```python
from build123d import *

# Parameters (mm, degrees)
BASE_FLANGE1_DEPTH                           = 19.5
SKETCH13_R                                   = 4
CUT_EXTRUDE6_DEPTH                           = 84.228219974
CUT_EXTRUDE7_DEPTH                           = 84.228219974
CUT_EXTRUDE7_DEPTH_BACK                      = 84.228219974
SKETCH33_R                                   = 8
CUT_EXTRUDE10_DEPTH                          = 10
SKETCH34_R                                   = 1.5
CUT_EXTRUDE11_DEPTH                          = 10
BOSS_EXTRUDE1_DEPTH                          = 3
TAB1_START                                   = -3
TAB1_DEPTH                                   = 3
CSK_FOR_M4_COUNTERSUNK_FLAT_HEAD_SCR_2_COUNT = 2
CSK_FOR_M4_COUNTERSUNK_FLAT_HEAD_SCR_2_PITCH = 39.597979746
CSK_FOR_M4_COUNTERSUNK_FLAT_HEAD_SCR_3_COUNT = 2
CSK_FOR_M4_COUNTERSUNK_FLAT_HEAD_SCR_3_PITCH = 56
CSK_FOR_M4_COUNTERSUNK_FLAT_HEAD_SCR_4_COUNT = 2
CSK_FOR_M4_COUNTERSUNK_FLAT_HEAD_SCR_4_PITCH = 39.597979746
SKETCH44_R                                   = 1.25
CUT_EXTRUDE13_DEPTH                          = 10
SKETCH45_R                                   = 1.25
CUT_EXTRUDE14_DEPTH                          = 10


# Read off the part's stored shape, not the designer's step: Tab1
# Sheet-metal steps are written as plain solids
with BuildPart() as part:
    # Sketch1 → Base-Flange1 (new, symmetric)
    with BuildSketch(Plane.XY):
        with BuildLine():
            Line((-28.21, 74.65), (-28.21, 2))
            ThreePointArc((-28.21, 2), (-27.624213562, 0.585786438), (-26.21, 0))
            Line((-26.21, 0), (26.21, 0))
            ThreePointArc((26.21, 0), (27.624213562, 0.585786438), (28.21, 2))
            Line((28.21, 2), (28.21, 74.65))
            Line((28.21, 74.65), (31.21, 74.65))
            Line((31.21, 74.65), (31.21, 2))
            ThreePointArc((31.21, 2), (29.745533906, -1.535533906), (26.21, -3))
            Line((26.21, -3), (-26.21, -3))
            ThreePointArc((-26.21, -3), (-29.745533906, -1.535533906), (-31.21, 2))
            Line((-31.21, 2), (-31.21, 74.65))
            Line((-31.21, 74.65), (-28.21, 74.65))
        make_face()
    extrude(amount=BASE_FLANGE1_DEPTH, both=True)

    # Sketch13 → Cut-Extrude6 (cut, through all)
    with BuildSketch(Plane(origin=(0, 0, 0), x_dir=(0, 0, -1), z_dir=(1, 0, 0))):
        with Locations((0, 32)):
            Circle(SKETCH13_R)
    extrude(amount=CUT_EXTRUDE6_DEPTH, mode=Mode.SUBTRACT)

    # Sketch15 → Cut-Extrude7 (cut, two sides: drawn at the far end of the back side and taken through both)
    with BuildSketch(Plane(origin=(0, 0, 0), x_dir=(0, 0, -1), z_dir=(1, 0, 0)).offset(-CUT_EXTRUDE7_DEPTH_BACK)):
        with BuildLine():
            Line((-19.5, 32), (-26.744382408, 32))
            Line((-26.744382408, 32), (-26.744382408, 87.632847334))
            Line((-26.744382408, 87.632847334), (26.744382408, 87.632847334))
            Line((26.744382408, 87.632847334), (26.744382408, 32))
            Line((26.744382408, 32), (19.5, 32))
            ThreePointArc((19.5, 32), (0, 51.5), (-19.5, 32))
        make_face()
        with BuildLine():
            Line((7.470480628, 19.147299148), (10, 14.795349466))
            ThreePointArc((10, 14.795349466), (10.176160856, 13.182152576), (9.097954318, 11.969342816))
            ThreePointArc((9.097954318, 11.969342816), (0, 10), (-9.097954318, 11.969342816))
            ThreePointArc((-9.097954318, 11.969342816), (-10.176160856, 13.182152576), (-10, 14.795349466))
            Line((-10, 14.795349466), (-7.470480628, 19.147299148))
            ThreePointArc((-7.470480628, 19.147299148), (-6.381394917, 20.037080634), (-4.975835097, 19.989959822))
            ThreePointArc((-4.975835097, 19.989959822), (0, 19), (4.975835097, 19.989959822))
            ThreePointArc((4.975835097, 19.989959822), (6.381394917, 20.037080634), (7.470480628, 19.147299148))
        make_face()
    extrude(amount=CUT_EXTRUDE7_DEPTH + CUT_EXTRUDE7_DEPTH_BACK, mode=Mode.SUBTRACT)

    # Sketch33 → Cut-Extrude10 (cut)
    with BuildSketch(Plane(origin=(-28.21, 0, 0), x_dir=(0, 0, -1), z_dir=(1, 0, 0))):
        with Locations((0, 32)):
            Circle(SKETCH33_R)
    extrude(amount=-CUT_EXTRUDE10_DEPTH, mode=Mode.SUBTRACT)

    # Sketch34 → Cut-Extrude11 (cut)
    with BuildSketch(Plane.ZY.offset(31.21)):
        with Locations((-11.490485194, 43.490485194)):
            Circle(SKETCH34_R)
        with Locations((11.490485194, 43.490485194)):
            Circle(SKETCH34_R)
        with Locations((11.490485194, 20.509514806)):
            Circle(SKETCH34_R)
        with Locations((-11.490485194, 20.509514806)):
            Circle(SKETCH34_R)
    extrude(amount=-CUT_EXTRUDE11_DEPTH, mode=Mode.SUBTRACT)

    # Sketch37 → Boss-Extrude1 (add)
    with BuildSketch(Plane.ZY.offset(31.21)):
        with BuildLine():
            Line((7.470480628, 19.147299148), (10, 14.795349466))
            ThreePointArc((10, 14.795349466), (10.176160856, 13.182152576), (9.097954318, 11.969342816))
            ThreePointArc((9.097954318, 11.969342816), (0, 10), (-9.097954318, 11.969342816))
            ThreePointArc((-9.097954318, 11.969342816), (-10.176160856, 13.182152576), (-10, 14.795349466))
            Line((-10, 14.795349466), (-7.470480628, 19.147299148))
            ThreePointArc((-7.470480628, 19.147299148), (-6.381394917, 20.037080634), (-4.975835097, 19.989959822))
            ThreePointArc((-4.975835097, 19.989959822), (0, 19), (4.975835097, 19.989959822))
            ThreePointArc((4.975835097, 19.989959822), (6.381394917, 20.037080634), (7.470480628, 19.147299148))
        make_face()
    extrude(amount=-BOSS_EXTRUDE1_DEPTH)

    # Tab1 outline → Tab1 (add)
    with BuildSketch(Plane.XZ.offset(3).offset(TAB1_START)):
        with BuildLine():
            Line((26.21, 19.5), (26.21, 23.195600876))
            ThreePointArc((26.21, 23.195600876), (0, 35), (-26.21, 23.195600876))
            Line((-26.21, 23.195600876), (-26.21, 19.5))
            Line((-26.21, 19.5), (26.21, 19.5))
        make_face()
        with BuildLine():
            Line((-26.21, -19.5), (-26.21, -23.195600876))
            ThreePointArc((-26.21, -23.195600876), (0, -35), (26.21, -23.195600876))
            Line((26.21, -23.195600876), (26.21, -19.5))
            Line((26.21, -19.5), (-26.21, -19.5))
        make_face()
    extrude(amount=TAB1_DEPTH)

    # Sketch42 → CSK for M4 Countersunk Flat Head Screw1 (revolve, cut)
    with BuildSketch(Plane(origin=(19.798989873, 0, -19.798989873), x_dir=(0, 0, 1), z_dir=(1, 0, 0))):
        Polygon((0, 0), (0, 3), (2.25, 3), (2.25, 2.45), (4.7, 0), align=None)
    csk_for_m4_countersunk_flat_head_screw1 = revolve(axis=Axis((19.798989873, 6.35, -19.798989873), (0, -1, 0)), mode=Mode.SUBTRACT)

    # CSK for M4 Countersunk Flat Head Scr 2: CSK for M4 Countersunk Flat Head Screw1 ×2
    with Locations(*[(-i * CSK_FOR_M4_COUNTERSUNK_FLAT_HEAD_SCR_2_PITCH, 0, 0) for i in range(1, CSK_FOR_M4_COUNTERSUNK_FLAT_HEAD_SCR_2_COUNT)]):
        add(csk_for_m4_countersunk_flat_head_screw1, mode=Mode.SUBTRACT)

    # CSK for M4 Countersunk Flat Head Scr 3: CSK for M4 Countersunk Flat Head Screw1 ×2
    with Locations(*[Vector(-0.7071067811865476, 0, 0.7071067811865476) * (i * CSK_FOR_M4_COUNTERSUNK_FLAT_HEAD_SCR_3_PITCH) for i in range(1, CSK_FOR_M4_COUNTERSUNK_FLAT_HEAD_SCR_3_COUNT)]):
        add(csk_for_m4_countersunk_flat_head_screw1, mode=Mode.SUBTRACT)

    # CSK for M4 Countersunk Flat Head Scr 4: CSK for M4 Countersunk Flat Head Screw1 ×2
    with Locations(*[(0, 0, i * CSK_FOR_M4_COUNTERSUNK_FLAT_HEAD_SCR_4_PITCH) for i in range(1, CSK_FOR_M4_COUNTERSUNK_FLAT_HEAD_SCR_4_COUNT)]):
        add(csk_for_m4_countersunk_flat_head_screw1, mode=Mode.SUBTRACT)

    # Sketch44 → Cut-Extrude13 (cut)
    with BuildSketch(Plane(origin=(0, 0, 0), x_dir=(1, 0, 0), z_dir=(0, 1, 0))):
        with Locations(Location((0, 25, 0), (0, 0, 270))):
            Circle(SKETCH44_R)
        with Locations(Location((12, 22, 0), (0, 0, 270))):
            Circle(SKETCH44_R)
        with Locations(Location((-12, 22, 0), (0, 0, 90))):
            Circle(SKETCH44_R)
        with Locations(Location((12, -22, 0), (0, 0, 90))):
            Circle(SKETCH44_R)
        with Locations(Location((0, -25, 0), (0, 0, 90))):
            Circle(SKETCH44_R)
        with Locations(Location((-12, -22, 0), (0, 0, 270))):
            Circle(SKETCH44_R)
        with BuildLine():
            Line((-11.5, 10.087120501), (-11.5, -10.087120501))
            ThreePointArc((-11.5, -10.087120501), (-10.88985573, -12.48068827), (-9.208333333, -14.290087376))
            ThreePointArc((-9.208333333, -14.290087376), (0, -17), (9.208333333, -14.290087376))
            ThreePointArc((9.208333333, -14.290087376), (10.88985573, -12.48068827), (11.5, -10.087120501))
            Line((11.5, -10.087120501), (11.5, 10.087120501))
            ThreePointArc((11.5, 10.087120501), (10.88985573, 12.48068827), (9.208333333, 14.290087376))
            ThreePointArc((9.208333333, 14.290087376), (0, 17), (-9.208333333, 14.290087376))
            ThreePointArc((-9.208333333, 14.290087376), (-10.88985573, 12.48068827), (-11.5, 10.087120501))
        make_face()
    extrude(amount=-CUT_EXTRUDE13_DEPTH, mode=Mode.SUBTRACT)

    # Sketch45 → Cut-Extrude14 (cut)
    with BuildSketch(Plane(origin=(31.21, 0, 0), x_dir=(0, 0, -1), z_dir=(1, 0, 0))):
        with Locations((-16, 7.5)):
            Circle(SKETCH45_R)
        with Locations((16, 7.5)):
            Circle(SKETCH45_R)
    extrude(amount=-CUT_EXTRUDE14_DEPTH, mode=Mode.SUBTRACT)


solid = part.part
```
Geometry: final body of the model. Coordinates: model frame, mm. A direction names the side the tool comes from. Coordinates: 2 decimals unless noted, no trailing zeros. Loops run counter-clockwise (first coordinate to the right, second up) from the corner with the lowest first, then second, coordinate; pieces in that order, holes last. Notation, with made-up numbers: (-16.5, -32) -> (1.5, -32) arc R22 ccw to (1.5, -23) -> close; hole circle Ø6 at (-3, 39.25). An arc over 180 degrees is marked (long way). Use a Markdown table: item, result. Add a question column.
(1) Pin query (flat end, axial travel): pin 1 Ø2 at (x, z) = (-20, -5.5) entering from +Y; pin 2 Ø4 at (y, z) = (7.5, 16) entering from +X; pin 3 Ø7 at (y, z) = (32, 0) entering from +X; pin 4 Ø2.5 at (y, z) = (-1.5, 3) entering from -X. Return the tip coordinate at first contact, or that it passes through.
(2) Section query C-C, the plane y = 26.5. Return loops of the section in (x, z).
(3) Line query: line 1 along X through (y, z) = (-0.8, -25); line 2 along X through (y, z) = (35, 19); line 3 along Y through (x, z) = (29.5, -1). Output: solid intervals per line, ascending.
(4) Mould query, pull axis X, two halves, no side actions, for faces 1 (the flat face through (-12, 0, 0)), 2 (the cylindrical face through (-29.731, 51.495, -0.429)), 3 (the flat face through (-31.21, 22, 0)). Classes: pulls with the +X half, pulls with the -X half, needs draft (parallel to the pull), parting line crosses it, or undercut.
(5) Section query B-B, the plane x = 0. Return loops of the section in (y, z).
(6) Access query for faces 4 (the cylindrical face through (-10.906, -1.479, 12.45)), 5 (the flat face through (-26.21, -1, 21)), 6 (the cylindrical face through (29.73, 6.28, -15.73)), 7 (the cylindrical face through (-29.689, 39.932, 1.041)), 8 (the flat face through (-26.21, -1, -21)). Directions: +Z, -Z, +X, -X, +Y, -Y. A direction counts if a zero-diameter tool reaches every point of the face in a straight line with its end or side. Return the directions, or none.
(7) Section query D-D, the plane z = -16. State how many separate pieces and enclosed holes the cut face has, plus the area to 3 significant figures.
(8) Section query A-A, the plane y = 7.5. Return loops of the section in (x, z).
Answer:
| question | item | result |
|---|---|---|
| 1 | pin 1 | stops at y = 0 |
| 1 | pin 2 | stops at x = 31.21 |
| 1 | pin 3 | passes through |
| 1 | pin 4 | stops at x = -30.68 |
| 2 | outline | (-31.21, -19.5) -> (-28.21, -19.5) -> (-28.21, -5.81) -> (-31.21, -5.81) -> close; (-31.21, 5.81) -> (-28.21, 5.81) -> (-28.21, 19.5) -> (-31.21, 19.5) -> close; (28.21, -19.5) -> (31.21, -19.5) -> (31.21, 19.5) -> (28.21, 19.5) -> close |
| 3 | line 1 | x = -24.49 to -1.25, 1.25 to 24.49 |
| 3 | line 2 | x = -31.21 to -28.21, 28.21 to 31.21 |
| 3 | line 3 | y = -1.77 to 10.02, 19.04 to 28.13, 35.87 to 51.47 |
| 4 | face 1 | undercut |
| 4 | face 2 | needs draft |
| 4 | face 3 | pulls with the -X half |
| 5 | outline | (-3, -35) -> (0, -35) -> (0, -26.25) -> (-3, -26.25) -> close; (-3, -23.75) -> (0, -23.75) -> (0, -17) -> (-3, -17) -> close; (-3, 17) -> (0, 17) -> (0, 23.75) -> (-3, 23.75) -> close; (-3, 26.25) -> (0, 26.25) -> (0, 35) -> (-3, 35) -> close |
| 6 | face 4 | +Y, -Y |
| 6 | face 5 | +Z, -X, +Y, -Y |
| 6 | face 6 | +X |
| 6 | face 7 | -X |
| 6 | face 8 | -Z, -X, +Y, -Y |
| 7 | separate pieces | 3 |
| 7 | enclosed holes | 0 |
| 7 | area | 389 mm^2 |
| 8 | outline | (-31.21, -19.5) -> (-28.21, -19.5) -> (-28.21, 19.5) -> (-31.21, 19.5) -> close; (28.21, -19.5) -> (31.21, -19.5) -> (31.21, -17.25) -> (28.21, -17.25) -> close; (28.21, -14.75) -> (31.21, -14.75) -> (31.21, 14.75) -> (28.21, 14.75) -> close; (28.21, 17.25) -> (31.21, 17.25) -> (31.21, 19.5) -> (28.21, 19.5) -> close |
